Could you check a few things on this model? Use its own coordinates, in mm. Give positions to 0.01 mm unless a question says otherwise; leave off trailing zeros. Write each loop counter-clockwise with the first axis right and the second up, starting at its lowest first coordinate (ties: lowest second). Pieces come first, ordered by that corner, then holes. Notation, with made-up numbers: (81.25, -6) - (97.25, -6) arc R32 ccw to (97.25, 27) - close; hole circle Ø9 at (-30, -16.5). An arc over 180 degrees is marked (long way). Answer as a JSON object with one key per item and string values. Group by question number.
```python
from build123d import *

# Parameters (mm, degrees)
BOSS_EXTRUDE1_DEPTH = 6


with BuildPart() as part:
    # Sketch1 → Boss-Extrude1 (new body)
    with BuildSketch(Plane(origin=(0, 0, 0), x_dir=(1, 0, 0), z_dir=(0, 1, 0))):
        with BuildLine():
            Line((-232, -140.040234189), (13.316058598, -140.040234189))
            Line((13.316058598, -140.040234189), (13.316058598, -231.040234189))
            Line((13.316058598, -231.040234189), (19.316058598, -231.040234189))
            Line((19.316058598, -231.040234189), (19.316058598, -140.040234189))
            Line((19.316058598, -140.040234189), (132, -140.040234189))
            ThreePointArc((132, -140.040234189), (202.864098928, -169.483310481), (231.999056434, -240.474644527))
            Line((231.999056434, -240.474644527), (149.958626336, -241.040376839))
            Line((149.958626336, -241.040376839), (150, -247.040234189))
            Line((150, -247.040234189), (100, -247.040234189))
            Line((100, -247.040234189), (100, -241.040234189))
            Line((100, -241.040234189), (-64, -241.040234189))
            Line((-64, -241.040234189), (-64, -246.040234189))
            Line((-64, -246.040234189), (-114, -246.040234189))
            Line((-114, -246.040234189), (-114, -240.040234189))
            Line((-114, -240.040234189), (-232, -240.040234189))
            Line((-232, -240.040234189), (-232, -140.040234189))
        make_face()
    extrude(amount=BOSS_EXTRUDE1_DEPTH)


solid = part.part
```
(1) I need wall thicknesses on L1, parallel to X at y = 1, z = 226; L2, parallel to X at y = 4.25, z = 238; L3, parallel to Z at x = 40, y = 0.95. Which ranges of each line are inside material? Lowest first, please.
(2) I want a section at A-A, the plane y = 1.35. Please give me the cut outline in (x, z).
(3) Will these pins go through, and if not, where does the flat tip stop? P1, Ø1.5, axis at y = 4, z = 182, coming from the +X side; P2, Ø1, axis at y = 2, z = 169.5, coming from the +X side; P3, Ø3, axis at x = -22.5, y = 2, coming from the +Z side.
(4) I want a section at C-C, the plane x = 50. Please give me the cut outline in (y, z), and give its area (3 significant figures).
(5) I want a section at D-D, the plane x = 186.5. Please give me the cut outline in (y, z).
(6) I want a section at B-B, the plane z = 203. Please give me the cut outline in (x, y), and give its area (3 significant figures).
Entries:
{
 "1": {"L1": "-232 to 13.32, 19.32 to 231.01", "L2": "-232 to 231.98", "L3": "140.04 to 241.04"},
 "2": {"outline": "(-232, 140.04) - (13.32, 140.04) - (13.32, 231.04) - (19.32, 231.04) - (19.32, 140.04) - (132, 140.04) arc R100 ccw to (232, 240.47) - (149.96, 241.04) - (150, 247.04) - (100, 247.04) - (100, 241.04) - (-64, 241.04) - (-64, 246.04) - (-114, 246.04) - (-114, 240.04) - (-232, 240.04) - close"},
 "3": {"P1": "x = 213.96", "P2": "x = 203.37", "P3": "z = 241.04"},
 "4": {"outline": "(0, 140.04) - (6, 140.04) - (6, 241.04) - (0, 241.04) - close", "area": "606 mm^2"},
 "5": {"outline": "(0, 156.2) - (6, 156.2) - (6, 240.79) - (0, 240.79) - close"},
 "6": {"outline": "(-232, 0) - (13.32, 0) - (13.32, 6) - (-232, 6) - close; (19.32, 0) - (224.89, 0) - (224.89, 6) - (19.32, 6) - close", "area": "2,710 mm^2"}
}
